Geometry check sheet. Reference: the model listing, model coordinates, mm. Face numbers are marked on the shaded views. Coordinates: 2 decimals unless noted, no trailing zeros. Write each loop counter-clockwise with the first axis right and the second up, starting at its lowest first coordinate (ties: lowest second). Pieces come first, ordered by that corner, then holes. Notation, with made-up numbers: (88, 87) -> (125, 87) arc R26 cw to (125, 103) -> close; hole circle Ø8 at (-35.5, 1). An arc over 180 degrees is marked (long way). Answer in a Markdown table with one row per item. Add a question column.
1. Cross-section at C-C on y = 2. Record the cut outline in (x, z), and give its area (3 significant figures).
2. Cross-section at A-A on x = 19.5. Record the cut outline in (y, z), and give its area (3 significant figures).
3. Mould release check, pull along X, two halves, no side actions. Record for the marked faces 1, 2 and 3: pulls with the +X half, pulls with the -X half, needs draft (parallel to the pull), parting line crosses it, or undercut.
4. Cross-section at B-B on z = -33. Record the cut outline in (x, y), and give its area (3 significant figures).
5. Cross-section at D-D on y = 4. Record the cut outline in (x, z).
6. Scan lines: L1, parallel to Y at x = 19.5, z = -30.5; L2, parallel to X at y = 2, z = -31.25; L3, parallel to X at y = 2, z = -26.75. Record each from-to range of solid material in increasing order. Write a range as from..to.
```python
from build123d import *

# Parameters (mm, degrees)
BOX001027045162_W     = 17
BOX001027045162_H     = 18
BOX001027045162_DEPTH = 16
CYLINDER208_R         = 1.4
CYLINDER208_DEPTH     = 30
BOX001027045158_W     = 33
BOX001027045158_H     = 16
BOX001027045158_DEPTH = 10
BOX001027045156_W     = 21
BOX001027045156_H     = 9.5
BOX001027045156_DEPTH = 10
CHAMFER018_SIZE       = 5
FILLET026_R           = 3


with BuildPart() as cube210:
    # Box001027045162 → Box001027045162 (new body)
    with BuildSketch(Plane(origin=(0, -8, -36), x_dir=(1, 0, 0), z_dir=(0, 0, 1))):
        with Locations((8.5, 9)):
            Rectangle(BOX001027045162_W, BOX001027045162_H)
    extrude(amount=BOX001027045162_DEPTH)


with BuildPart() as cylinder252:
    # Cylinder208 → Cylinder208 (new body)
    with BuildSketch(Plane(origin=(19.5, 2, -45), x_dir=(1, 0, 0), z_dir=(0, 0, 1))):
        Circle(CYLINDER208_R)
    extrude(amount=CYLINDER208_DEPTH)


with BuildPart() as cube206:
    # Box001027045158 → Box001027045158 (new body)
    with BuildSketch(Plane(origin=(0, -7, -44), x_dir=(1, 0, 0), z_dir=(0, 0, 1))):
        with Locations((16.5, 8)):
            Rectangle(BOX001027045158_W, BOX001027045158_H)
    extrude(amount=BOX001027045158_DEPTH)


with BuildPart() as adjust_block:
    # Box001027045156 → Box001027045156 (new body)
    with BuildSketch(Plane(origin=(20, -2.5, -42), x_dir=(1, 0, 0), z_dir=(0, 0, 1))):
        with Locations((10.5, 4.75)):
            Rectangle(BOX001027045156_W, BOX001027045156_H)
    extrude(amount=BOX001027045156_DEPTH)

    # Chamfer018
    chamfer018_edges = [adjust_block.edges().sort_by_distance(p)[0] for p in [
        (20, 2.25, -32),
        (41, 2.25, -32),
    ]]
    chamfer(chamfer018_edges, length=CHAMFER018_SIZE)

    # Fillet026
    fillet026_edges = [adjust_block.edges().sort_by_distance(p)[0] for p in [
        (25, 2.25, -32),
        (36, 2.25, -32),
    ]]
    fillet(fillet026_edges, radius=FILLET026_R)


with BuildPart() as adjust_block_1:
    # Fillet026 placement: moved
    add(adjust_block.part.moved(Location((-11, -2, 7))))

    # Cut181: cut Cube206
    add(cube206.part, mode=Mode.SUBTRACT)

    # Cut183: cut Cylinder252
    add(cylinder252.part, mode=Mode.SUBTRACT)

    # Cut188: cut Cube210
    add(cube210.part, mode=Mode.SUBTRACT)


solid = adjust_block_1.part
```
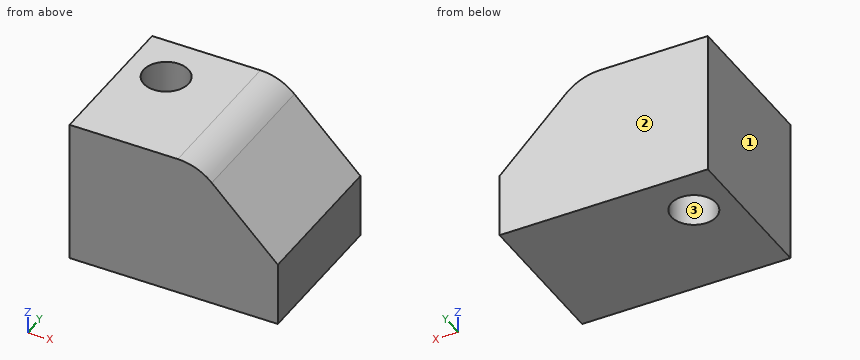
Results found:
| question | item | result |
|---|---|---|
| 1 | outline | (17, -34) -> (18.1, -34) -> (18.1, -25) -> (17, -25) -> close; (20.9, -34) -> (30, -34) -> (30, -30) -> (25.88, -25.88) arc R3 ccw to (23.76, -25) -> (20.9, -25) -> close |
| 1 | area | 79.1 mm^2 |
| 2 | outline | (-4.5, -34) -> (0.6, -34) -> (0.6, -25) -> (-4.5, -25) -> close; (3.4, -34) -> (5, -34) -> (5, -25) -> (3.4, -25) -> close |
| 2 | area | 60.3 mm^2 |
| 3 | face 1 | pulls with the -X half |
| 3 | face 2 | needs draft |
| 3 | face 3 | undercut |
| 4 | outline | (17, -4.5) -> (30, -4.5) -> (30, 5) -> (17, 5) -> close; hole circle Ø2.8 at (19.5, 2) |
| 4 | area | 117 mm^2 |
| 5 | outline | (17, -34) -> (30, -34) -> (30, -30) -> (25.88, -25.88) arc R3 ccw to (23.76, -25) -> (17, -25) -> close |
| 6 | L1 | y = -4.5..0.6, 3.4..5 |
| 6 | L2 | x = 17..18.1, 20.9..30 |
| 6 | L3 | x = 17..18.1, 20.9..26.75 |
